from build123d import *

# Parameters (mm, degrees)
SKETCH1_W           = 120
SKETCH1_H           = 40
BOSS_EXTRUDE1_DEPTH = 3
SKETCH2_R           = 7.45
SKETCH2_R_2         = 9.525
SKETCH2_R_3         = 3.175
CUT_EXTRUDE1_DEPTH  = 4
SKETCH4_W           = 10
SKETCH4_H           = 3
BOSS_EXTRUDE2_DEPTH = 3
SKETCH5_W           = 3
SKETCH5_H           = 10
CUT_EXTRUDE2_DEPTH  = 4


with BuildPart() as part:
    # Sketch1 → Boss-Extrude1 (new body)
    with BuildSketch(Plane(origin=(0, 0, 0), x_dir=(1, 0, 0), z_dir=(0, 1, 0))):
        Rectangle(SKETCH1_W, SKETCH1_H)
    extrude(amount=BOSS_EXTRUDE1_DEPTH)

    # Sketch2 → Cut-Extrude1 (cut, through all)
    with BuildSketch(Plane(origin=(0, 3, 0), x_dir=(1, 0, 0), z_dir=(0, 1, 0))):
        with Locations((45, 0)):
            Circle(SKETCH2_R)
        with Locations((-45, 0)):
            Circle(SKETCH2_R)
        Circle(SKETCH2_R_2)
        with Locations((10.375, 10.375)):
            Circle(SKETCH2_R_3)
        with Locations((10.375, -10.375)):
            Circle(SKETCH2_R_3)
        with Locations((-10.375, -10.375)):
            Circle(SKETCH2_R_3)
        with Locations((-10.375, 10.375)):
            Circle(SKETCH2_R_3)
    extrude(amount=-CUT_EXTRUDE1_DEPTH, mode=Mode.SUBTRACT)

    # Sketch4 → Boss-Extrude2 (add)
    with BuildSketch(Plane(origin=(0, 3, 0), x_dir=(1, 0, 0), z_dir=(0, 1, 0))):
        with Locations((15, 21.5)):
            Rectangle(SKETCH4_W, SKETCH4_H)
        with Locations((35, 21.5)):
            Rectangle(SKETCH4_W, SKETCH4_H)
        with Locations((55, 21.5)):
            Rectangle(SKETCH4_W, SKETCH4_H)
        with Locations((-55, 21.5)):
            Rectangle(SKETCH4_W, SKETCH4_H)
        with Locations((-35, 21.5)):
            Rectangle(SKETCH4_W, SKETCH4_H)
        with Locations((-15, 21.5)):
            Rectangle(SKETCH4_W, SKETCH4_H)
        with Locations((-15, -21.5)):
            Rectangle(SKETCH4_W, SKETCH4_H)
        with Locations((-35, -21.5)):
            Rectangle(SKETCH4_W, SKETCH4_H)
        with Locations((-55, -21.5)):
            Rectangle(SKETCH4_W, SKETCH4_H)
        with Locations((55, -21.5)):
            Rectangle(SKETCH4_W, SKETCH4_H)
        with Locations((35, -21.5)):
            Rectangle(SKETCH4_W, SKETCH4_H)
        with Locations((15, -21.5)):
            Rectangle(SKETCH4_W, SKETCH4_H)
    extrude(amount=-BOSS_EXTRUDE2_DEPTH)

    # Sketch5 → Cut-Extrude2 (cut, through all)
    with BuildSketch(Plane(origin=(0, 3, 0), x_dir=(1, 0, 0), z_dir=(0, 1, 0))):
        with Locations((58.5, 10)):
            Rectangle(SKETCH5_W, SKETCH5_H)
        with Locations((58.5, -10)):
            Rectangle(SKETCH5_W, SKETCH5_H)
    cut_extrude2 = extrude(amount=-CUT_EXTRUDE2_DEPTH, mode=Mode.SUBTRACT)

    # Mirror1: Cut-Extrude2 across plane
    add(cut_extrude2.mirror(Plane(origin=(0, 0, 0), x_dir=(0, 0, 1), z_dir=(1, 0, 0))), mode=Mode.SUBTRACT)


solid = part.part
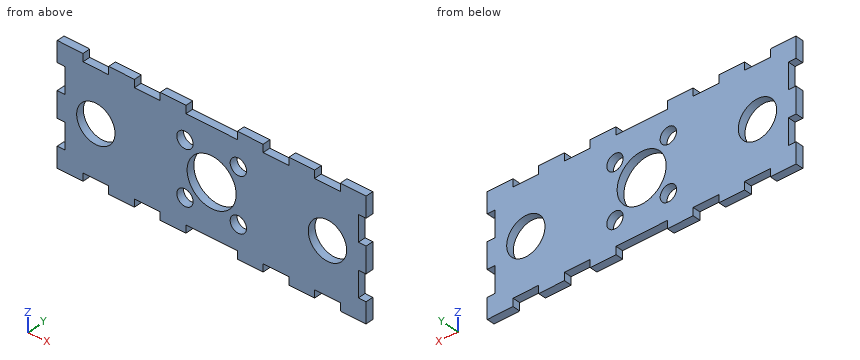
Build history of the part. All positions in model axes, mm. Coordinates: 2 decimals unless noted, no trailing zeros. Order: outer loops, then holes, each group sorted by start corner. A loop starts at its lowest first (then second) coordinate and runs counter-clockwise, first axis right, second up. Notation, with made-up numbers: (-28.5, 11.25) -> (27.5, 11.25) arc R20 ccw to (27.5, 17.25) -> close; hole circle Ø7 at (8, 61.5). An arc over 180 degrees is marked (long way). One line per item, written item: value.
(1) Slice it at B-B, the plane z = 0. List the corners of the cut face in (x, y) (3 decimals), plus the area to 3 significant figures.
Checked values:
outline: (-60, 0) -> (-52.45, 0) -> (-52.45, 3) -> (-60, 3) -> close; (-37.55, 0) -> (-9.525, 0) -> (-9.525, 3) -> (-37.55, 3) -> close; (9.525, 0) -> (37.55, 0) -> (37.55, 3) -> (9.525, 3) -> close; (52.45, 0) -> (60, 0) -> (60, 3) -> (52.45, 3) -> close
area: 213 mm2
(2) Slice it at D-D, the plane y = 1.65. Count the separate pieces of the cut face and the enclosed holes in it, plus the area to 3 significant figures.
Checked values:
separate pieces: 1
enclosed holes: 7
area: 4,280 mm2
(3) Probe line 1 (X direction, y = 2.1, z = 0) (3 decimals); line 2 (X direction, y = 0.55, z = -21); line 3 (Z direction, x = 13, y = 0.5). List the from-to ranges inside material, lowest first. Write a range as [from, to].
Checked values:
line 1: [-60, -52.45], [-37.55, -9.525], [9.525, 37.55], [52.45, 60]
line 2: [-60, -50], [-40, -30], [-20, -10], [10, 20], [30, 40], [50, 60]
line 3: [-23, -12.16], [-8.59, 8.59], [12.16, 23]
(4) Slice it at C-C, the plane x = 45. List the corners of the cut face in (y, z).
Checked values:
outline: (0, -20) -> (3, -20) -> (3, -7.45) -> (0, -7.45) -> close; (0, 7.45) -> (3, 7.45) -> (3, 20) -> (0, 20) -> close
(5) Drop a flat-ended pin along its axis: pin 1 Ø19.5 at (x, z) = (45, 0) entering from +Y. Give the stop position or say it passes through.
Checked values:
pin 1: y = 3
(6) Slice it at A-A, the plane x = 0. List the corners of the cut face in (y, z) (3 decimals).
Checked values:
outline: (0, -20) -> (3, -20) -> (3, -9.525) -> (0, -9.525) -> close; (0, 9.525) -> (3, 9.525) -> (3, 20) -> (0, 20) -> close
